from build123d import *

# Parameters (mm, degrees)
F0_R     = 4
F1_DEPTH = 7
F2_R     = 1.5
F3_DEPTH = 3.8
F4_W     = 10
F4_H     = 2
F5_DEPTH = 7
F6_R     = 0.8
F7_DEPTH = 4.001


with BuildPart() as f1:
    # F0 (on Top) → F1 (new body, symmetric)
    with BuildSketch(Plane.XY):
        Circle(F0_R)
    extrude(amount=F1_DEPTH, both=True)

    # F2 (on face) → F3 (cut)
    with BuildSketch(Plane.XY.offset(7)):
        Circle(F2_R)
    extrude(amount=-F3_DEPTH, mode=Mode.SUBTRACT)

    # F4 (on face) → F5 (cut)
    with BuildSketch(Plane(origin=(0, 0, -7), x_dir=(1, 0, 0), z_dir=(0, 0, -1))):
        Rectangle(F4_W, F4_H)
    extrude(amount=-F5_DEPTH, mode=Mode.SUBTRACT)

    # F6 (on Front) → F7 (cut, through all)
    with BuildSketch(Plane.XZ):
        with Locations((0, 5.1)):
            Circle(F6_R)
    extrude(amount=F7_DEPTH, mode=Mode.SUBTRACT)


solid = f1.part
Source: CAD feature listing. Evaluate the final solid. Frame: model axes, mm. A direction names the side the tool comes from. Round coordinates to 2 decimals unless told otherwise and drop trailing zeros. Loops run counter-clockwise (first coordinate to the right, second up) from the corner with the lowest first, then second, coordinate; pieces in that order, holes last. Notation, with made-up numbers: (46.25, 35) - (65.25, 35) arc R29 cw to (65.25, 69) - close; hole circle Ø10 at (26.5, -26). An arc over 180 degrees is marked (long way). Write item = value, one per line. Start each with the question number.
(1) Ray query, line 1 along Y through (x, z) = (0, 6.25); line 2 along Z through (x, y) = (-2.5, 0.75); line 3 along Z through (x, y) = (0.5, -0.75). Return the intervals inside material, ascending. Write a range as from..to.
(2) Section query D-D, the plane x = -2.5. Output: boundary loops of the cut face in (y, z), plus the area to 3 significant figures.
(3) Section query A-A, the plane x = 0. Output: boundary loops of the cut face in (y, z), plus the area to 3 significant figures.
(4) Section query C-C, the plane z = -5. Output: boundary loops of the cut face in (x, y).
(5) Set-up query: faces 4 (the face through (-0.8, -2.6, 5.1)), 5 (the face through (0, 0, 3.2)), 6 (the face through (0, 1, -4)), 7 (the face through (0, 2, -7)). Return all of +Z, -Z, +X, -X, +Y, -Y with unobstructed straight access to the full face (end or side cutting, diameter ignored); none if empty.
(6) Pin query (flat end, axial travel): pin 1 (3 mm diameter, centred on y = 2, z = 3, fed in from -X); pin 2 (1.5 mm diameter, centred on y = -2, z = -5, fed in from +X). Return the tip coordinate at first contact, or that it passes through.
(7) Pull-direction query (X, two-part tool) for faces 1 (the face through (-0.195, 1.487, 5.127)), 2 (the face through (3.695, -1.532, 0.098)), 3 (the face through (2, 0, 7)); classes: +X half, -X half, draft (parallel to the pull), parting line (faces both ways), or undercut.
(8) Section query B-B, the plane y = 0. Output: boundary loops of the cut face in (x, z), plus the area to 3 significant figures.
Conclusion:
q1.line_1 = -4..-1.5, 1.5..4
q1.line_2 = 0..7
q1.line_3 = 0..3.2
q2.outline = (-3.12, -7) - (-1, -7) - (-1, 0) - (1, 0) - (1, -7) - (3.12, -7) - (3.12, 7) - (-3.12, 7) - close
q2.area = 73.4 mm2
q3.outline = (-4, -7) - (-1, -7) - (-1, 0) - (1, 0) - (1, -7) - (4, -7) - (4, 7) - (1.5, 7) - (1.5, 3.2) - (-1.5, 3.2) - (-1.5, 4.3) - (-4, 4.3) - close; (-4, 5.9) - (-1.5, 5.9) - (-1.5, 7) - (-4, 7) - close
q3.area = 82.6 mm2
q4.outline = (-3.87, -1) arc R4 ccw to (3.87, -1) - close; (-3.87, 1) - (3.87, 1) arc R4 ccw to start
q5.face_4 = -Y
q5.face_5 = +Z
q5.face_6 = -Z, +X, -X
q5.face_7 = -Z, +X, -X, +Y, -Y
q6.pin_1 = -3.97
q6.pin_2 = 3.8
q7.face_1 = undercut
q7.face_2 = parting line
q7.face_3 = draft
q8.outline = (-4, 0) - (4, 0) - (4, 7) - (1.5, 7) - (1.5, 3.2) - (-1.5, 3.2) - (-1.5, 7) - (-4, 7) - close
q8.area = 44.6 mm2
